Build history of the part. All positions in model axes, mm. Face numbers are marked on the shaded views. A direction names the side the tool comes from. Round coordinates to 2 decimals unless told otherwise and drop trailing zeros. Loops run counter-clockwise (first coordinate to the right, second up) from the corner with the lowest first, then second, coordinate; pieces in that order, holes last. Notation, with made-up numbers: (6, -4.75) -> (58, -4.75) arc R16 cw to (58, 0.25) -> close; hole circle Ø2 at (21, 53). An arc over 180 degrees is marked (long way). Put each result on its own line as item: value. Start each with the question number.
Item 1: Tool access for the marked faces 5, 6, 7 and 8: list every direction of +Z, -Z, +X, -X, +Y, -Y with a clear straight run to the whole face (end or side of a thin tool).
Item 2: Drill centre lines: probe 1 along Z at (x, y) = (4.5, -3); probe 2 along Z at (x, y) = (0.75, 2); probe 3 along X at (y, z) = (-11, 2.5). Where is each one in solid material? Low to high. Write a range as [from, to].
Item 3: Flat gauge pins, fed straight in: pin 1 Ø0.8 at (x, z) = (1, 4) entering from -Y; pin 2 Ø1 at (x, y) = (-4, 1.5) entering from -Z; pin 3 Ø2.5 at (x, z) = (3.5, -1) entering from +Y. Where does each tip first touch, or does it go through?
Item 4: Cut at C-C, the plane x = 5. List the corners of the cut face in (y, z), plus the area to 3 significant figures.
Item 5: Cut at A-A, the plane z = -1.25. List the corners of the cut face in (x, y).
Item 6: Pull direction Z, two halves, no side cores. Call the marked faces 1, 2, 3 and 4: +Z half, -Z half, draft (parallel to the pull), parting line (faces both ways), or undercut.
Item 7: Cut at B-B, the plane z = 3.5. List the corners of the cut face in (x, y).
Item 8: Cut at D-D, the plane y = 3.5. List the corners of the cut face in (x, z), plus the area to 3 significant figures.
```python
from build123d import *

# Parameters (mm, degrees)
F1_DEPTH      = 4.2
F2_DEPTH      = 2.5
F3_DEPTH      = 5
F3_DEPTH_BACK = 5
F4_W          = 5
F4_H          = 5
F5_DEPTH      = 4
F5_DEPTH_BACK = 4
F6_SIZE       = 2
F7_W          = 4
F7_H          = 2.5
F8_DEPTH      = 25
F9_R          = 2
F11_DEPTH     = 1
F13_DEPTH     = 1
F14_T1_DEPTH  = 16.8989794856


# Not quite as in the source:
# - a fillet or chamfer that OpenCascade refuses, or shapes differently, is made with other operations: its cross-section is extruded or revolved along the edge and cut away or added


with BuildPart() as f1:
    # F0 (on Top) → F1 (new body)
    with BuildSketch(Plane.XY):
        with BuildLine():
            ThreePointArc((6, 14.5), (0, 20.5), (-6, 14.5))
            Line((-6, 14.5), (-3.65, 14.5))
            ThreePointArc((-3.65, 14.5), (-2.5809397513, 17.0809397513), (0, 18.15))
            ThreePointArc((0, 18.15), (2.5809397513, 17.0809397513), (3.65, 14.5))
            Line((3.65, 14.5), (6, 14.5))
        make_face()
        with BuildLine():
            Line((6, -6.5), (-6, -6.5))
            Line((-6, -6.5), (-6, -10.5))
            ThreePointArc((-6, -10.5), (-4.8284271247, -13.3284271247), (-2, -14.5))
            Line((-2, -14.5), (-2, -10.5))
            Line((-2, -10.5), (0, -10.5))
            Line((0, -10.5), (2, -10.5))
            Line((2, -10.5), (2, -14.5))
            ThreePointArc((2, -14.5), (4.8284271247, -13.3284271247), (6, -10.5))
            Line((6, -10.5), (6, -6.5))
        make_face()
        with BuildLine():
            Line((-3.65, 14.5), (-6, 14.5))
            Line((-6, 14.5), (-6, -6.5))
            Line((-6, -6.5), (6, -6.5))
            Line((6, -6.5), (6, 14.5))
            Line((6, 14.5), (3.65, 14.5))
            ThreePointArc((3.65, 14.5), (3.6264789057, 14.0862963062), (3.5562187692, 13.6779245377))
            Line((3.5562187692, 13.6779245377), (1.9871117367, -0.0766868897))
            ThreePointArc((1.9871117367, -0.0766868897), (1.3316580306, -1.3422087286), (0, -1.85))
            ThreePointArc((0, -1.85), (-1.3316580225, -1.3422087358), (-1.9871117342, -0.0766869112))
            Line((-1.9871117342, -0.0766869112), (-3.5562187692, 13.6779245377))
            ThreePointArc((-3.5562187692, 13.6779245377), (-3.6264789057, 14.0862963062), (-3.65, 14.5))
        make_face()
    extrude(amount=F1_DEPTH)

    # F0 (on Top) → F2 (join)
    with BuildSketch(Plane.XY):
        with BuildLine():
            ThreePointArc((0, 10.85), (-2.2717751388, 11.6431594866), (-3.5562187692, 13.6779245377))
            Line((-3.5562187692, 13.6779245377), (-1.9871117342, -0.0766869112))
            ThreePointArc((-1.9871117342, -0.0766869112), (-1.4922087358, 1.4816580225), (0, 2.15))
            Line((0, 2.15), (0, 10.85))
        make_face()
        with BuildLine():
            ThreePointArc((3.5562187692, 13.6779245377), (2.2717751388, 11.6431594866), (0, 10.85))
            Line((0, 10.85), (0, 2.15))
            ThreePointArc((0, 2.15), (1.4142135624, 1.5642135624), (2, 0.15))
            ThreePointArc((2, 0.15), (1.9967753346, 0.0364735127), (1.9871117367, -0.0766868897))
            Line((1.9871117367, -0.0766868897), (3.5562187692, 13.6779245377))
        make_face()
        with BuildLine():
            ThreePointArc((0, 2.15), (-1.4922087358, 1.4816580225), (-1.9871117342, -0.0766869112))
            ThreePointArc((-1.9871117342, -0.0766869112), (-1.3316580225, -1.3422087358), (0, -1.85))
            Line((0, -1.85), (0, 2.15))
        make_face()
        with BuildLine():
            ThreePointArc((2, 0.15), (1.4142135624, 1.5642135624), (0, 2.15))
            Line((0, 2.15), (0, -1.85))
            ThreePointArc((0, -1.85), (1.3316580306, -1.3422087286), (1.9871117367, -0.0766868897))
            ThreePointArc((1.9871117367, -0.0766868897), (1.9967753346, 0.0364735127), (2, 0.15))
        make_face()
    extrude(amount=F2_DEPTH)

    # F0 (on Top) → F3 (join, two sides)
    with BuildSketch(Plane.XY) as f3_sk:
        with BuildLine():
            Line((6, -6.5), (-6, -6.5))
            Line((-6, -6.5), (-6, -10.5))
            ThreePointArc((-6, -10.5), (-4.8284271247, -13.3284271247), (-2, -14.5))
            Line((-2, -14.5), (-2, -10.5))
            Line((-2, -10.5), (0, -10.5))
            Line((0, -10.5), (2, -10.5))
            Line((2, -10.5), (2, -14.5))
            ThreePointArc((2, -14.5), (4.8284271247, -13.3284271247), (6, -10.5))
            Line((6, -10.5), (6, -6.5))
        make_face()
    extrude(amount=F3_DEPTH)
    extrude(f3_sk.sketch, amount=-F3_DEPTH_BACK)

    # F4 (on face) → F5 (cut, two sides)
    with BuildSketch(Plane(origin=(0, -6.5, 0), x_dir=(-1, 0, 0), z_dir=(0, 1, 0))) as f5_sk:
        Rectangle(F4_W, F4_H)
    extrude(amount=-F5_DEPTH, mode=Mode.SUBTRACT)
    extrude(f5_sk.sketch, amount=F5_DEPTH_BACK, mode=Mode.SUBTRACT)

    # F6
    f6_edges = [f1.edges().sort_by_distance(p)[0] for p in [
        (0, -2.5, 2.5),
    ]]
    chamfer(f6_edges, length=F6_SIZE)

    # F7 (on face) → F8 (cut)
    with BuildSketch(Plane.XZ.offset(10.5)):
        with Locations((0, -3.75)):
            Rectangle(F7_W, F7_H)
    extrude(amount=-F8_DEPTH, mode=Mode.SUBTRACT)

    # F9
    f9_edges = [f1.edges().sort_by_distance(p)[0] for p in [
        (4, -6.5, -5),
        (-4, -6.5, -5),
    ]]
    fillet(f9_edges, radius=F9_R)

    # F10 (on face) → F11 (join)
    with BuildSketch(Plane.YZ.offset(-2)):
        with BuildLine():
            Line((-6.5, -2.5), (-10.5, -2.5))
            Line((-10.5, -2.5), (-10.5, -5))
            Line((-10.5, -5), (-8.5, -5))
            ThreePointArc((-8.5, -5), (-7.0857864376, -4.4142135624), (-6.5, -3))
            Line((-6.5, -3), (-6.5, -2.5))
        make_face()
    extrude(amount=F11_DEPTH)

    # F12 (on face) → F13 (join)
    with BuildSketch(Plane(origin=(2, 0, 0), x_dir=(0, -1, 0), z_dir=(-1, 0, 0))):
        with BuildLine():
            Line((10.5, -5), (10.5, -2.5))
            Line((10.5, -2.5), (6.5, -2.5))
            Line((6.5, -2.5), (6.5, -3))
            ThreePointArc((6.5, -3), (7.0857864376, -4.4142135624), (8.5, -5))
            Line((8.5, -5), (10.5, -5))
        make_face()
    extrude(amount=F13_DEPTH)

    # F14: fillet of radius 1 on 1 edges, made by hand

    # F14_s2 → F14_t1 (cut)
    with BuildSketch(Plane.YZ.offset(-8.4494897428)):
        with BuildLine():
            ThreePointArc((-6.5, 4.2), (-6.8473403651, 4.7745966692), (-7.4797958971, 5))
            Line((-7.4797958971, 5), (-6.5, 5))
            Line((-6.5, 5), (-6.5, 4.2))
        make_face()
    extrude(amount=F14_T1_DEPTH, mode=Mode.SUBTRACT)


solid = f1.part
```
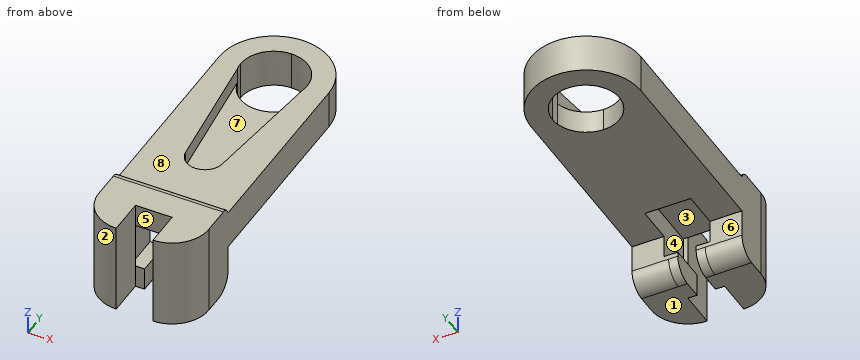
Reply:
1. face 5: +Z, -Z, -Y
1. face 6: -Z, +X, -X, +Y
1. face 7: +Z
1. face 8: +Z, +X, -X, +Y
2. probe 1: z = [0, 4.2]
2. probe 2: z = [0, 2.5]
2. probe 3: x = [-5.97, -2], [2, 5.97]
3. pin 1: stops at y = -10.5
3. pin 2: stops at z = 0
3. pin 3: stops at y = 19.83
4. outline: (-13.15, -5) -> (-8.5, -5) arc R2 ccw to (-6.5, -3) -> (-6.5, 0) -> (17.82, 0) -> (17.82, 4.2) -> (-6.5, 4.2) arc R1 ccw to (-7.48, 5) -> (-13.15, 5) -> close
4. area: 168 mm^2
5. outline: (-6, -10.5) arc R4 ccw to (-2, -14.5) -> (-2, -10.5) -> (-2.5, -10.5) -> (-2.5, -6.5) -> (-6, -6.5) -> close; (2, -14.5) arc R4 ccw to (6, -10.5) -> (6, -6.5) -> (2.5, -6.5) -> (2.5, -10.5) -> (2, -10.5) -> close
6. face 1: -Z half
6. face 2: draft
6. face 3: undercut
6. face 4: undercut
7. outline: (-6, -10.5) arc R4 ccw to (-2, -14.5) -> (-2, -10.5) -> (2, -10.5) -> (2, -14.5) arc R4 ccw to (6, -10.5) -> (6, 14.5) arc R6 ccw to (-6, 14.5) -> close; hole (-3.56, 13.68) -> (-1.99, -0.08) arc R2 ccw to (1.99, -0.08) -> (3.56, 13.68) arc R3.65 ccw (long way) to start
8. outline: (-6, 0) -> (6, 0) -> (6, 4.2) -> (2.4, 4.2) -> (2.4, 2.5) -> (-2.4, 2.5) -> (-2.4, 4.2) -> (-6, 4.2) -> close
8. area: 42.3 mm^2
